Geometry check sheet. Reference: the model listing, model coordinates, mm. Face numbers are marked on the shaded views. A direction names the side the tool comes from. Round coordinates to 2 decimals unless told otherwise and drop trailing zeros. Order: outer loops, then holes, each group sorted by start corner. A loop starts at its lowest first (then second) coordinate and runs counter-clockwise, first axis right, second up.
(1) Sectioned sample at A-A (x = 0). Record the boundary of the cut face in (y, z).
(2) Set-up check for the marked faces 1 and 2: record each of +Z, -Z, +X, -X, +Y, -Y from which the full face is reachable in a straight line by a thin tool's end or side.
(3) Material ranges on line 1 along X through (y, z) = (2.5, 2.5); line 2 along Y through (x, z) = (8.75, 3.05); line 3 along Z through (x, y) = (7, 5.5), recorded low to high.
(4) Sectioned sample at C-C (x = 5.5). Record the boundary of the cut face in (y, z).
(5) Sectioned sample at B-B (y = 2.5). Record the boundary of the cut face in (x, z), plus the area to 3 significant figures.
(6) Go/stop test with a flat-tipped pin: pin 1 (7 mm diameter, centred on x = 0, y = 2.5, fed in from -Z). Record where the tip stops, or that it passes through.
(7) Sectioned sample at D-D (z = -1.5). Record the boundary of the cut face in (x, y), plus the area to 3 significant figures.
(8) Release check for a two-part mould opening along Y. For the marked faces 3, 4, 5 and 6 record: +Y half, -Y half, draft (parallel to the pull), parting line (faces both ways), or undercut.
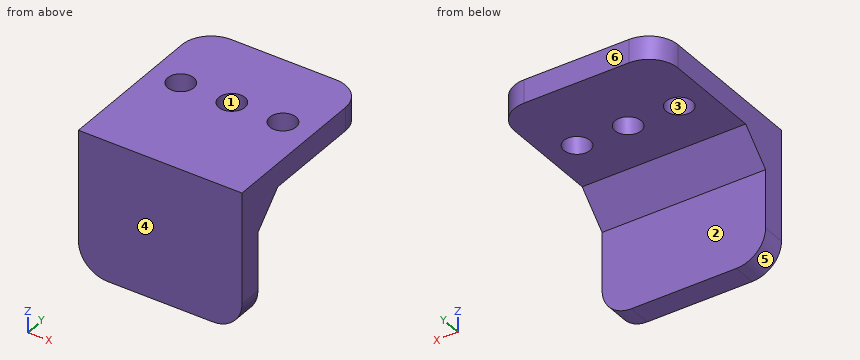
Autodesk Inventor part; units mm, degrees
ref_plane "YZ Plane" through (0, 0, 0) normal (1, 0, 0) x (0, 1, 0)
ref_plane "XZ Plane" through (0, 0, 0) normal (0, 1, 0) x (-1, 0, 0)
ref_plane "XY Plane" through (0, 0, 0) normal (0, 0, 1) x (1, 0, 0)
sketch "Sketch1" plane through (0, 0, 0) normal (0, 0, 1) x (1, 0, 0)
  line L0 (-14, 15.5) -> (14, 15.5)
  line L1 (14, 15.5) -> (14, -15.5)
  line L2 (14, -15.5) -> (-14, -15.5)
  line L3 (-14, -15.5) -> (-14, 15.5)
  line L4 (-14, 15.5) -> (14, -15.5) construction
  line L5 (14, 15.5) -> (-14, -15.5) construction
  point P0 (0, 0)
  dimension "d0" = 28
  dimension "d1" = 31
extrude "Extrusion1" add sketch "Sketch1" along normal blind 4
sketch "Sketch2" plane through (0, 0, 4) normal (0, 0, 1) x (1, 0, 0)
  line L0 (-14, -15.5) -> (14, -15.5)
  point P0 (0, 2.5)
  point P1 (-8.75, 2.5)
  point P2 (8.75, 2.5)
  dimension "d7" = 8.75
  dimension "d8" = 8.75
  dimension "d19" = 18
  dimension "d20" = 18
  dimension "d21" = 18
hole "Hole1" at (0, 2.5, 4) at (-8.75, 2.5, 4) at (8.75, 2.5, 4) direction (0, 0, -1) diameter 4.5 end through all
sketch "Sketch3" plane through (0, 0, 0) normal (0, 0, -1) x (-1, 0, 0)
  line L0 (14, -15.5) -> (-14, -15.5)
  line L1 (14, 15.5) -> (14, -15.5)
  line L2 (-14, -15.5) -> (14, -15.5)
  line L3 (14, -15.5) -> (14, -11.5)
  line L4 (14, -11.5) -> (-14, -11.5)
  line L5 (-14, -11.5) -> (-14, -15.5)
  point P0 (0, 0)
  dimension "d16" = 4
extrude "Extrusion2" add sketch "Sketch3" along normal blind 20
chamfer "Chamfer1" distance 5 angle 45 1 edges at (0, -11.5, 0)
fillet "Fillet1" radius 5 4 edges at (14, 15.5, 2) (-14, 15.5, 2) (14, -13.5, -20) (-14, -13.5, -20)
properties part number "BLTouch"
Answer below:
1. outline: (-15.5, -20) - (-11.5, -20) - (-11.5, -5) - (-6.5, 0) - (0.25, 0) - (0.25, 4) - (-15.5, 4) - close; (4.75, 0) - (15.5, 0) - (15.5, 4) - (4.75, 4) - close
2. face 1: +Z, -Z
2. face 2: -Z, +X, -X, +Y
3. line 1: x = -14 to -11, -6.5 to -2.25, 2.25 to 6.5, 11 to 14
3. line 2: y = -15.5 to 0.25, 4.75 to 15.5
3. line 3: z = 0 to 4
4. outline: (-15.5, -20) - (-11.5, -20) - (-11.5, -5) - (-6.5, 0) - (15.5, 0) - (15.5, 4) - (-15.5, 4) - close
5. outline: (-14, 0) - (-11, 0) - (-11, 4) - (-14, 4) - close; (-6.5, 0) - (-2.25, 0) - (-2.25, 4) - (-6.5, 4) - close; (2.25, 0) - (6.5, 0) - (6.5, 4) - (2.25, 4) - close; (11, 0) - (14, 0) - (14, 4) - (11, 4) - close
5. area: 58.0 mm2
6. pin 1: stops at z = 0
7. outline: (-14, -15.5) - (14, -15.5) - (14, -8) - (-14, -8) - close
7. area: 210 mm2
8. face 3: undercut
8. face 4: -Y half
8. face 5: draft
8. face 6: +Y half
